Can you work these out from the model? Positions are in its coordinate system, mm. A direction names the side the tool comes from. Round coordinates to 2 decimals unless told otherwise and drop trailing zeros. Loops run counter-clockwise (first coordinate to the right, second up) from the corner with the lowest first, then second, coordinate; pieces in that order, holes last. Notation, with made-up numbers: (-5.5, 32.5) - (11.5, 32.5) arc R29 cw to (11.5, 54.5) - close; hole circle Ø8 at (72.25, -3). An arc over 180 degrees is marked (long way). Answer as CSV lines item,"result".
```python
from build123d import *

# Parameters (mm, degrees)
SKETCH1_R               = 16.25
BOSS_EXTRUDE1_DEPTH     = 2
SKETCH2_R               = 15
BOSS_EXTRUDE2_DEPTH     = 6
BOSS_EXTRUDE3_START     = 7
SKETCH3_R               = 15
BOSS_EXTRUDE3_DEPTH     = 7
CUT_EXTRUDE1_DEPTH      = 28.443123
CUT_EXTRUDE1_DEPTH_BACK = 8
SKETCH4_R               = 2.9
CUT_EXTRUDE2_DEPTH      = 25.33361872
CUT_EXTRUDE2_DEPTH_BACK = 25.33361872
SKETCH5_R               = 2.2


with BuildPart() as part:
    # Sketch1 → Boss-Extrude1 (new body)
    with BuildSketch(Plane(origin=(0, 0, 0), x_dir=(1, 0, 0), z_dir=(0, 1, 0))):
        with Locations(Location((0, 0, 0), (0, 0, 270))):
            Circle(SKETCH1_R)
    extrude(amount=BOSS_EXTRUDE1_DEPTH)

    # Sketch2 → Boss-Extrude2 (add)
    with BuildSketch(Plane.XZ):
        with Locations(Location((0, 0, 0), (0, 0, 270))):
            Circle(SKETCH2_R)
    extrude(amount=BOSS_EXTRUDE2_DEPTH)

    # Sketch3 → Boss-Extrude3 (add)
    with BuildSketch(Plane(origin=(0, 2, 0), x_dir=(1, 0, 0), z_dir=(0, 1, 0)).offset(BOSS_EXTRUDE3_START)):
        with Locations(Location((0, 0, 0), (0, 0, 90))):
            Circle(SKETCH3_R)
    extrude(amount=-BOSS_EXTRUDE3_DEPTH)

    # Sketch4 → Cut-Extrude1 (cut, two sides: drawn at the far end of the back side and taken through both)
    with BuildSketch(Plane(origin=(0, 9, 0), x_dir=(1, 0, 0), z_dir=(0, 1, 0)).offset(-CUT_EXTRUDE1_DEPTH_BACK)):
        with Locations(Location((0, 7.5, 0), (0, 0, 90))):
            Circle(SKETCH4_R)
        with Locations(Location((0, -7.5, 0), (0, 0, 90))):
            Circle(SKETCH4_R)
    extrude(amount=CUT_EXTRUDE1_DEPTH + CUT_EXTRUDE1_DEPTH_BACK, mode=Mode.SUBTRACT)

    # Sketch5 → Cut-Extrude2 (cut, two sides: drawn at the far end of the back side and taken through both)
    with BuildSketch(Plane(origin=(0, 1, 0), x_dir=(1, 0, 0), z_dir=(0, 1, 0)).offset(-CUT_EXTRUDE2_DEPTH_BACK)):
        with Locations(Location((0, 7.5, 0), (0, 0, 270))):
            Circle(SKETCH5_R)
        with Locations(Location((0, -7.5, 0), (0, 0, 270))):
            Circle(SKETCH5_R)
    extrude(amount=CUT_EXTRUDE2_DEPTH + CUT_EXTRUDE2_DEPTH_BACK, mode=Mode.SUBTRACT)


solid = part.part
```
Q1. We'd pull the mould along Z, two halves only. Please class faces 1 (the flat face through (-11, 0, 11)), 2 (the cylindrical face through (-0.843, -2.549, 9.532)), 3 (the cylindrical face through (-0.66, 5.549, 14.985)): pulls with the +Z half, pulls with the -Z half, needs draft (parallel to the pull), parting line crosses it, or undercut.
Checks:
face 1,"needs draft"
face 2,"undercut"
face 3,"parting line crosses it"
Q2. Imagine slicing it at C-C (y = 6.25). Write out the boundary of the cut face in (x, z), then the cut area to 3 significant figures.
Checks:
outline,"circle Ø30 at (0, 0); hole circle Ø5.8 at (0, -7.5); hole circle Ø5.8 at (0, 7.5)"
area,"654 mm²"
Q3. Imagine slicing it at B-B (z = -7.5). Write out the boundary of the cut face in (x, y).
Checks:
outline,"(-14.42, 0) - (-12.99, 0) - (-12.99, -6) - (-2.2, -6) - (-2.2, 1) - (-2.9, 1) - (-2.9, 9) - (-12.99, 9) - (-12.99, 2) - (-14.42, 2) - close; (2.2, -6) - (12.99, -6) - (12.99, 0) - (14.42, 0) - (14.42, 2) - (12.99, 2) - (12.99, 9) - (2.9, 9) - (2.9, 1) - (2.2, 1) - close"
Q4. Imagine slicing it at A-A (x = 0). Write out the boundary of the cut face in (y, z).
Checks:
outline,"(-6, -15) - (0, -15) - (0, -16.25) - (2, -16.25) - (2, -15) - (9, -15) - (9, -10.4) - (1, -10.4) - (1, -9.7) - (-6, -9.7) - close; (-6, -5.3) - (1, -5.3) - (1, -4.6) - (9, -4.6) - (9, 4.6) - (1, 4.6) - (1, 5.3) - (-6, 5.3) - close; (-6, 9.7) - (1, 9.7) - (1, 10.4) - (9, 10.4) - (9, 15) - (2, 15) - (2, 16.25) - (0, 16.25) - (0, 15) - (-6, 15) - close"
Q5. On a 3-axis mill with a long thin cutter (end or side, diameter ignored), from which of +Z, -Z, +X, -X, +Y, -Y can I reach the whole of each face in a straight line? I mean faces 4 (the cylindrical face through (0.66, -2.958, 14.985)), 5 (the flat face through (0, 9, 0)), 6 (the flat face through (-2, 1, -9)). Say none if no direction works.
Checks:
face 4,"-Y"
face 5,"+Z, -Z, +X, -X, +Y"
face 6,"+Y"
Q6. If I drill on line 1 along Y through (x, z) = (5, 15); line 2 along X through (y, z) = (-3, -7.5); line 3 along X through (y, z) = (7, -7.5), over which ranges is the centre line in solid material (lowest first)? Write a range as [from, to].
Checks:
line 1,"[0, 2]"
line 2,"[-12.99, -2.2], [2.2, 12.99]"
line 3,"[-12.99, -2.9], [2.9, 12.99]"
Q7. I'm going to push flat-ended pins straight in: pin 1 Ø1.5 at (y, z) = (6.5, -6) entering from -X; pin 2 Ø8 at (x, y) = (9, 0.5) entering from -Z; pin 3 Ø5 at (x, z) = (0, -7.5) entering from +Y. Where does each tip first touch, or does it pass through?
Checks:
pin 1,"x = -14.05"
pin 2,"z = -15.46"
pin 3,"y = 1"
Q8. Imagine slicing it at D-D (z = 0). Write out the boundary of the cut face in (x, y).
Checks:
outline,"(-16.25, 0) - (-15, 0) - (-15, -6) - (15, -6) - (15, 0) - (16.25, 0) - (16.25, 2) - (15, 2) - (15, 9) - (-15, 9) - (-15, 2) - (-16.25, 2) - close"
